from build123d import *

# Parameters (mm, degrees)
SKETCH_1_W          = 18
SKETCH_1_H          = 17
EXTRUDE_1_DEPTH     = 6
EXTRUDE_2_DEPTH     = 6
SKETCH_8_R          = 1.35
CUT_EXTRUDE_4_DEPTH = 5
SKETCH_9_R          = 2
CUT_EXTRUDE_5_DEPTH = 10
SKETCH_10_W         = 20
SKETCH_10_H         = 8
CUT_EXTRUDE_6_DEPTH = 10
FILLET_1_R          = 3


with BuildPart() as part:
    # 草图1 → 凸台-拉伸1 (new body)
    with BuildSketch(Plane.XY):
        Rectangle(SKETCH_1_W, SKETCH_1_H)
    extrude(amount=EXTRUDE_1_DEPTH)

    # 草图6 → 凸台-拉伸2 (add)
    with BuildSketch(Plane(origin=(0, 0, 0), x_dir=(-1, 0, 0), z_dir=(0, 0, -1))):
        Polygon((-9, 8.5), (-14, 8.5), (-14, -3.5), (-20, -3.5), (-20, -8.5), (-9, -8.5), align=None)
        Polygon((20, -8.5), (20, -3.5), (14, -3.5), (14, 8.5), (9, 8.5), (9, -8.5), align=None)
    extrude(amount=-EXTRUDE_2_DEPTH)

    # 草图8 → 切除-拉伸4 (cut)
    with BuildSketch(Plane(origin=(0, -3.5, 0), x_dir=(1, 0, 0), z_dir=(0, 1, 0))):
        with Locations(Location((17, -3, 0), (0, 0, 180))):
            Circle(SKETCH_8_R)
        with Locations((-17, -3)):
            Circle(SKETCH_8_R)
    extrude(amount=-CUT_EXTRUDE_4_DEPTH, mode=Mode.SUBTRACT)

    # 草图9 → 切除-拉伸5 (cut)
    with BuildSketch(Plane.XY.offset(6)):
        with Locations((-6, 4.5)):
            Circle(SKETCH_9_R)
        with Locations(Location((6, 4.5, 0), (0, 0, 180))):
            Circle(SKETCH_9_R)
    extrude(amount=-CUT_EXTRUDE_5_DEPTH, mode=Mode.SUBTRACT)

    # 草图10 → 切除-拉伸6 (cut)
    with BuildSketch(Plane.XY.offset(6)):
        with Locations((0, -4.5)):
            Rectangle(SKETCH_10_W, SKETCH_10_H)
    extrude(amount=-CUT_EXTRUDE_6_DEPTH, mode=Mode.SUBTRACT)

    # 圆角1
    fillet_1_edges = [part.edges().sort_by_distance(p)[0] for p in [
        (14, 8.5, 3),
        (-14, 8.5, 3),
        (-10, -8.5, 3),
        (-10, -0.5, 3),
        (10, -0.5, 3),
        (10, -8.5, 3),
    ]]
    fillet(fillet_1_edges, radius=FILLET_1_R)


solid = part.part
Verification items for the finished model (mm, model axes). A direction names the side the tool comes from. Round coordinates to 2 decimals unless told otherwise and drop trailing zeros. Loops run counter-clockwise (first coordinate to the right, second up) from the corner with the lowest first, then second, coordinate; pieces in that order, holes last. Notation, with made-up numbers: (76, 43.25) - (96, 43.25) arc R25 ccw to (96, 59.25) - close; hole circle Ø11 at (25, 65). An arc over 180 degrees is marked (long way). Answer in a Markdown table with one row per item. Add a question column.
Q1. Section check D-D on y = 4.5. Enter the section's corners in (x, z).
Q2. Material ranges on line 1 (Z direction, x = 17, y = -5.1); line 2 (Y direction, x = -6, z = 3.85); line 3 (X direction, y = 6, z = 3.3), recorded low to high.
Q3. Gauge pin test, flat ends, axial feed: pin 1 (1 mm diameter, centred on x = 10.5, z = 5, fed in from -Y); pin 2 (10 mm diameter, centred on x = -1.5, y = -4.5, fed in from +Z). Record the tip position at first contact, or that the pin passes through.
Q4. Release check for a two-part mould opening along X. For faces 4 (the face through (9.1, -1.36, 2.96)), 5 (the face through (-15.67, -8.5, 2.29)), 6 (the face through (20, -6, 3)), 7 (the face through (-20, -6, 3)) record: pulls with the +X half, pulls with the -X half, needs draft (parallel to the pull), parting line crosses it, or undercut.
Q5. Section check C-C on z = 4.8. Enter the section's corners in (x, y).
Q6. Section check A-A on z = 3. Enter the section's corners in (x, y).
Q7. Tool access check on faces 1 (the face through (-14, 1, 3)), 2 (the face through (0, -0.5, 3)), 3 (the face through (15.6, -3.5, 2.3)). Record the directions out of +Z, -Z, +X, -X, +Y, -Y that give a thin tool (end or side, any length) a straight path to the whole face; none if there is none.
Q8. Section check B-B on x = 17. Enter the section's corners in (y, z).
Found:
| question | item | result |
|---|---|---|
| 1 | outline | (-14, 0) - (-8, 0) - (-8, 6) - (-14, 6) - close; (-4, 0) - (4, 0) - (4, 6) - (-4, 6) - close; (8, 0) - (14, 0) - (14, 6) - (8, 6) - close |
| 2 | line 1 | z = 0 to 1.65, 4.35 to 6 |
| 2 | line 2 | y = -0.5 to 2.5, 6.5 to 8.5 |
| 2 | line 3 | x = -13.96 to -7.32, -4.68 to 4.68, 7.32 to 13.96 |
| 3 | pin 1 | stops at y = -7.74 |
| 3 | pin 2 | stops at z = 6 |
| 4 | face 4 | undercut |
| 4 | face 5 | needs draft |
| 4 | face 6 | pulls with the +X half |
| 4 | face 7 | pulls with the -X half |
| 5 | outline | (-20, -8.5) - (-13, -8.5) arc R3 ccw to (-10, -5.5) - (-10, -3.5) arc R3 cw to (-7, -0.5) - (7, -0.5) arc R3 cw to (10, -3.5) - (10, -5.5) arc R3 ccw to (13, -8.5) - (20, -8.5) - (20, -3.5) - (14, -3.5) - (14, 5.5) arc R3 ccw to (11, 8.5) - (-11, 8.5) arc R3 ccw to (-14, 5.5) - (-14, -3.5) - (-20, -3.5) - close; hole circle Ø4 at (-6, 4.5); hole circle Ø4 at (6, 4.5) |
| 6 | outline | (-20, -8.5) - (-18.35, -8.5) - (-18.35, -3.5) - (-20, -3.5) - close; (-15.65, -8.5) - (-13, -8.5) arc R3 ccw to (-10, -5.5) - (-10, -3.5) arc R3 cw to (-7, -0.5) - (7, -0.5) arc R3 cw to (10, -3.5) - (10, -5.5) arc R3 ccw to (13, -8.5) - (15.65, -8.5) - (15.65, -3.5) - (14, -3.5) - (14, 5.5) arc R3 ccw to (11, 8.5) - (-11, 8.5) arc R3 ccw to (-14, 5.5) - (-14, -3.5) - (-15.65, -3.5) - close; (18.35, -8.5) - (20, -8.5) - (20, -3.5) - (18.35, -3.5) - close; hole circle Ø4 at (-6, 4.5); hole circle Ø4 at (6, 4.5) |
| 7 | face 1 | +Z, -Z, -X, +Y |
| 7 | face 2 | +Z, -Z, -Y |
| 7 | face 3 | +Z, -Z, +X, +Y |
| 8 | outline | (-8.5, 0) - (-3.5, 0) - (-3.5, 1.65) - (-8.5, 1.65) - close; (-8.5, 4.35) - (-3.5, 4.35) - (-3.5, 6) - (-8.5, 6) - close |
